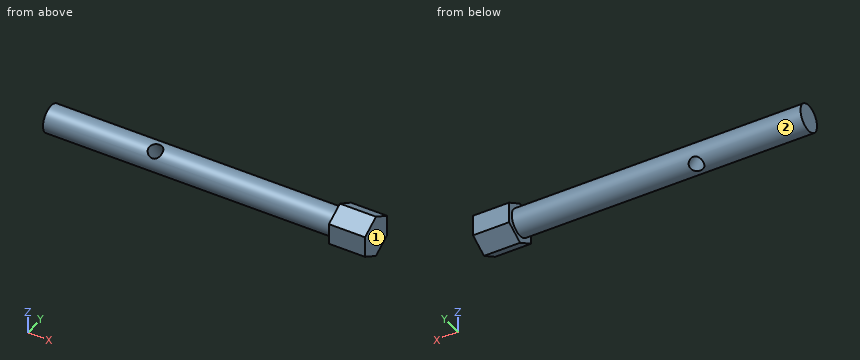
Autodesk Inventor part; units mm, degrees
ref_plane "YZ Plane" through (0, 0, 0) normal (1, 0, 0) x (0, 1, 0)
ref_plane "XZ Plane" through (0, 0, 0) normal (0, 1, 0) x (-1, 0, 0)
ref_plane "XY Plane" through (0, 0, 0) normal (0, 0, 1) x (1, 0, 0)
sketch "Sketch1" plane through (0, 0, 0) normal (1, 0, 0) x (0, 1, 0)
  circle A0 centre (0, 0) radius 4.7625
  dimension "d0" = 9.525
extrude "Extrusion1" add sketch "Sketch1" along normal blind 101.6
sketch "Sketch2" plane through (101.6, 0, 0) normal (1, 0, 0) x (0, 0, -1)
  circle A0 centre (0, 0) radius 4.7625
  line L0 (3.6662, 6.35) -> (7.3323, 0)
  line L1 (7.3323, 0) -> (3.6662, -6.35)
  line L2 (3.6662, -6.35) -> (-3.6662, -6.35)
  line L3 (-3.6662, -6.35) -> (-7.3323, 0)
  line L4 (-7.3323, 0) -> (-3.6662, 6.35)
  line L5 (-3.6662, 6.35) -> (3.6662, 6.35)
  dimension "d3" = 12.7
extrude "Extrusion2" add sketch "Sketch2" along normal blind 12.7 contours A0 | L0 L1 L2 L3 L4 L5
sketch "Sketch3" plane through (114.3, 0, -7.3323) normal (0, 0.5, -0.866) x (-1, 0, 0)
  circle A0 centre (76.2, 3.6662) radius 2.4384
  line L0 (12.7, 7.3323) -> (76.2, 7.3323) construction
  line L1 (76.2, 7.3323) -> (76.2, 3.6662) construction
  line L2 (76.2, 3.6662) -> (76.2, 0) construction
  line L3 (76.2, 0) -> (12.7, 0) construction
  point P0 (114.3, 3.6662)
  dimension "d6" = 4.8768
  dimension "d9" = 63.5
extrude "Extrusion3" cut sketch "Sketch3" against normal through all
properties part number "Shovel_RollerDriveAxle" material "Aluminum-6061-AHC"
The model under review builds one solid part; all positions refer to its coordinate system, in mm. Face numbers are marked on the shaded views. A direction names the side the tool comes from. Coordinates: 2 decimals unless noted, no trailing zeros. Write each loop counter-clockwise with the first axis right and the second up, starting at its lowest first coordinate (ties: lowest second). Pieces come first, ordered by that corner, then holes. Notation, with made-up numbers: (39.5, -38.75) - (90.5, -38.75) arc R26 cw to (90.5, -13.75) - close; hole circle Ø2 at (-19.5, 1). An arc over 180 degrees is marked (long way). Answer in a Markdown table with one row per item. Add a question column.
Q1. Clearance check with flat-ended pins moving along their axes: pin 1 (2 mm diameter, centred on x = 81, y = -3.5, fed in from +Z); pin 2 (6 mm diameter, centred on x = 65, y = 3, fed in from +Z); pin 3 (1 mm diameter, centred on x = 55, z = 5.5, fed in from +Y); pin 4 (3 mm diameter, centred on x = 12, y = -3, fed in from +Z). State where each tip first meets the part, or that it passes through.
Q2. Consider section A-A on x = 77. Give the boundary of the cut face in (y, z) (1 decimal).
Q3. To check wall thickness, follow line 1 along X through (y, z) = (-2.5, 3.75); line 2 along X through (y, z) = (-6, 2); line 3 along Z through (x, y) = (25, -0.25). State the ranges of each line that lie inside material, in increasing order. Write a range as from..to.
Q4. Consider section B-B on z = -6. Give the boundary of the cut face in (x, y), then the cut area to 3 significant figures.
Q5. For the marked faces 1 and 2, list the 3-axis set-ups (+Z, -Z, +X, -X, +Y, -Y) from which the entire face can be reached by the end or side of a thin tool; tool diameter is ignored.
Answers below:
| question | item | result |
|---|---|---|
| 1 | pin 1 | z = 4.05 |
| 1 | pin 2 | z = 4.76 |
| 1 | pin 3 | through |
| 1 | pin 4 | z = 4.52 |
| 2 | outline | circle Ø9.5 at (0, 0) |
| 3 | line 1 | 0..35.68, 40.52..114.3 |
| 3 | line 2 | 101.6..114.3 |
| 3 | line 3 | -4.76..4.76 |
| 4 | outline | (101.6, -2.31) - (114.3, -2.31) - (114.3, 2.31) - (101.6, 2.31) - close |
| 4 | area | 58.6 mm² |
| 5 | face 1 | +Z, -Z, +X, +Y, -Y |
| 5 | face 2 | -X |
